CAD build for the part. Positions are in the model's coordinates, mm. Round coordinates to 2 decimals unless told otherwise and drop trailing zeros. Write each loop counter-clockwise with the first axis right and the second up, starting at its lowest first coordinate (ties: lowest second). Pieces come first, ordered by that corner, then holes. Notation, with made-up numbers: (-35, 72.5) - (11, 72.5) arc R15 cw to (11, 85.5) - close; hole circle Ø4 at (56, -22). An arc over 180 degrees is marked (long way). Use one line per item in the form item = value. Start each with the question number.
Item 1: Band-saw the part on B-B, the plane y = 2.05. Give the number of separate pieces and of enclosed holes in the cut face, and give its area (3 significant figures).
Item 2: Band-saw the part on A-A, the plane x = 109. List the corners of the cut face in (y, z).
Item 3: Pull direction X, two halves, no side cores. Call faces 1 (the cylindrical face through (184.154, 1.479, -159.628)), 2 (the flat face through (118, 0, -101)): +X half, -X half, draft (parallel to the pull), parting line (faces both ways), or undercut.
Item 4: Pin check, flat tips, straight feed: pin 1 (10.5 mm diameter, centred on x = 192.5, z = -157, fed in from +Y); pin 2 (23 mm diameter, centred on x = 172, z = -177, fed in from -Y). Stop position of each tip, or through.
Item 5: Drill centre lines: L1, parallel to Z at x = 192.5, y = 1.7; L2, parallel to X at y = 1.4, z = -170; L3, parallel to Z at x = 88.5, y = 1.15. Where is each one in solid material? Low to high.
Item 6: Band-saw the part on C-C, the plane x = 221. List the corners of the cut face in (y, z).
from build123d import *

# Parameters (mm, degrees)
SKETCH1_W             = 240
SKETCH1_H             = 200
BOSS_EXTRUDE1_DEPTH   = 3
M16_CLEARANCE_HOLE1_D = 17.5
M22_CLEARANCE_HOLE1_D = 23


with BuildPart() as part:
    # Sketch1 → Boss-Extrude1 (new body)
    with BuildSketch(Plane(origin=(0, 0, 0), x_dir=(1, 0, 0), z_dir=(0, 1, 0))):
        with Locations((120, 100)):
            Rectangle(SKETCH1_W, SKETCH1_H)
    extrude(amount=BOSS_EXTRUDE1_DEPTH)

    # M16 Clearance Hole1 (through all)
    with Locations(Plane(origin=(0, 3, 0), x_dir=(1, 0, 0), z_dir=(0, 1, 0))):
        with Locations((19, 157), (47.5, 177), (67, 157), (88.5, 177), (109, 157), (129.5, 177), (150, 157), (172, 177), (192.5, 157)):
            Hole(M16_CLEARANCE_HOLE1_D / 2)

    # M22 Clearance Hole1 (through all)
    with Locations(Plane(origin=(0, 3, 0), x_dir=(1, 0, 0), z_dir=(0, 1, 0))):
        with Locations((221, 167)):
            Hole(M22_CLEARANCE_HOLE1_D / 2)


solid = part.part
Determined:
q1.separate_pieces = 1
q1.enclosed_holes = 10
q1.area = 45,400 mm²
q2.outline = (0, -200) - (3, -200) - (3, -165.75) - (0, -165.75) - close; (0, -148.25) - (3, -148.25) - (3, 0) - (0, 0) - close
q3.face_1 = undercut
q3.face_2 = draft
q4.pin_1 = through
q4.pin_2 = 0
q5.L1 = -200 to -165.75, -148.25 to 0
q5.L2 = 0 to 42.25, 52.75 to 83.25, 93.75 to 124.25, 134.75 to 166.75, 177.25 to 209.9, 232.1 to 240
q5.L3 = -200 to -185.75, -168.25 to 0
q6.outline = (0, -200) - (3, -200) - (3, -178.5) - (0, -178.5) - close; (0, -155.5) - (3, -155.5) - (3, 0) - (0, 0) - close
